Model file for the job. Use its own axes, mm. A direction names the side the tool comes from. Coordinates: 2 decimals unless noted, no trailing zeros. Write each loop counter-clockwise with the first axis right and the second up, starting at its lowest first coordinate (ties: lowest second). Pieces come first, ordered by that corner, then holes.
Q1. Band-saw the part on C-C, the plane z = -32. Write the cut outline in (x, y).
Q2. Band-saw the part on D-D, the plane z = 7.5. Write the cut outline in (x, y).
Q3. Pin check, flat tips, straight feed: P1, Ø1.5, axis at x = 22, y = 17, coming from the -Z side; P2, Ø8, axis at x = 26.5, y = -3, coming from the -Z side; P3, Ø9, axis at x = 7, z = -11.5, coming from the +Y side. Stop position of each tip, or through.
Q4. Drill centre lines: probe 1 along Y at (x, z) = (0, -36); probe 2 along Y at (x, z) = (30, 17.5); probe 3 along Z at (x, y) = (-14, -12). Where is each one in solid material? Low to high.
Q5. Band-saw the part on A-A, the plane y = 14. Write the cut outline in (x, z).
Q6. Which spindle directions (+Z, -Z, +X, -X, +Y, -Y) get a long thin tool onto all of the face, cutting with end or side? Do faces 4 (the flat face through (0, 20, -35)), 5 (the flat face through (-40, -25, 10)), 6 (the flat face through (0, -5, -15)), 7 (the cylindrical face through (0.651, -8.043, -34.93)). Say none if no direction does.
Q7. Band-saw the part on B-B, the plane x = 0. Write the cut outline in (y, z).
Q8. Pull direction Z, two halves, no side cores. Call faces 1 (the flat face through (50, 0, 10)), 2 (the flat face through (0, 13, -30)), 3 (the flat face through (0, 0, -40)): released by +Z, released by -Z, zero draft, split by the parting line, or undercut.
from build123d import *

# Parameters (mm, degrees)
EXTRUDE_1_DEPTH = 20
EXTRUDE_2_DEPTH = 10
SKETCH_3_R      = 5
EXTRUDE_3_DEPTH = 10


with BuildPart() as part:
    # 草圖1 → 填料-伸長1 (new body)
    with BuildSketch(Plane.XY):
        with BuildLine():
            Line((50, 40), (-50, 40))
            Line((-50, 40), (-50, 35))
            Line((-50, 35), (-30, 35))
            ThreePointArc((-30, 35), (-25, 30), (-30, 25))
            Line((-30, 25), (-50, 25))
            Line((-50, 25), (-50, -25))
            Line((-50, -25), (-30, -25))
            ThreePointArc((-30, -25), (-25, -30), (-30, -35))
            Line((-30, -35), (-50, -35))
            Line((-50, -35), (-50, -40))
            Line((-50, -40), (50, -40))
            Line((50, -40), (50, -35))
            Line((50, -35), (30, -35))
            ThreePointArc((30, -35), (25, -30), (30, -25))
            Line((30, -25), (50, -25))
            Line((50, -25), (50, 25))
            Line((50, 25), (30, 25))
            ThreePointArc((30, 25), (25, 30), (30, 35))
            Line((30, 35), (50, 35))
            Line((50, 35), (50, 40))
        make_face()
    extrude(amount=EXTRUDE_1_DEPTH)

    # 草圖2 → 填料-伸長2 (add)
    with BuildSketch(Plane(origin=(0, -5, 0), x_dir=(-1, 0, 0), z_dir=(0, -1, 0))):
        with BuildLine():
            ThreePointArc((15, 10), (17.928932188, 2.928932188), (25, 0))
            Line((25, 0), (-25, 0))
            ThreePointArc((-25, 0), (-17.928932188, 2.928932188), (-15, 10))
            Line((-15, 10), (-15, 30))
            Line((-15, 30), (15, 30))
            Line((15, 30), (15, 10))
        make_face()
    extrude(amount=-EXTRUDE_2_DEPTH)

    # 草圖3 → 填料-伸長3 (add)
    with BuildSketch(Plane(origin=(0, 0, -30), x_dir=(-1, 0, 0), z_dir=(0, 0, -1))):
        with BuildLine():
            Line((-15, 20), (15, 20))
            Line((15, 20), (15, -13))
            ThreePointArc((15, -13), (0, -20), (-15, -13))
            Line((-15, -13), (-15, 20))
        make_face()
        with Locations((0, -13)):
            Circle(SKETCH_3_R, mode=Mode.SUBTRACT)
    extrude(amount=EXTRUDE_3_DEPTH)


solid = part.part
Answer sheet:
1. outline: (-15, -13) arc R19.57 ccw to (15, -13) - (15, 20) - (-15, 20) - close; hole circle Ø10 at (0, -13)
2. outline: (-50, -40) - (50, -40) - (50, -35) - (30, -35) arc R5 cw to (30, -25) - (50, -25) - (50, 25) - (30, 25) arc R5 cw to (30, 35) - (50, 35) - (50, 40) - (-50, 40) - (-50, 35) - (-30, 35) arc R5 cw to (-30, 25) - (-50, 25) - (-50, -25) - (-30, -25) arc R5 cw to (-30, -35) - (-50, -35) - close
3. P1: stops at z = 0
3. P2: stops at z = -0.32
3. P3: stops at y = 5
4. probe 1: y = -20 to -18, -8 to 20
4. probe 2: y = -40 to -35, -25 to 25, 35 to 40
4. probe 3: z = -40 to -30, 0 to 20
5. outline: (-50, 0) - (50, 0) - (50, 20) - (-50, 20) - close; (-15, -40) - (15, -40) - (15, -30) - (-15, -30) - close
6. face 4: -Z, +X, -X, +Y
6. face 5: +Z, -Z, -X
6. face 6: +X, -X, -Y
6. face 7: -Z
7. outline: (-40, 0) - (-5, 0) - (-5, -30) - (-8, -30) - (-8, -40) - (20, -40) - (20, -30) - (5, -30) - (5, 0) - (40, 0) - (40, 20) - (-40, 20) - close; (-20, -40) - (-18, -40) - (-18, -30) - (-20, -30) - close
8. face 1: zero draft
8. face 2: undercut
8. face 3: released by -Z
